```python
from build123d import *

# Parameters (mm, degrees)
F0_R         = 12.5
F0_R_2       = 10.9
F3_W         = 620
F3_H         = 800
F4_DEPTH     = 1.6
F5_R         = 15
F6_R         = 15
F7_W         = 558.6059093475
F7_H         = 742.6531389356
F8_DEPTH     = 15
F9_W         = 530.512617901
F9_H         = 715.3386492282
F10_DEPTH    = 15
F11_R        = 5
F12_T1_DEPTH = 10
F12_S5_W     = 5.1
F12_S5_H     = 5.1
F12_T6_DEPTH = 5.1


# Not quite as in the source:
# - a fillet or chamfer that OpenCascade refuses, or shapes differently, is made with other operations: its cross-section is extruded or revolved along the edge and cut away or added


with BuildPart() as f2:
    # F2: sweep along a path in F1
    with BuildLine(Plane.XZ) as f2_path:
        Line((0, 0), (0, 800))
        ThreePointArc((0, 800), (29.2893218813, 870.7106781187), (100, 900))
        Line((100, 900), (450, 900))
        ThreePointArc((450, 900), (520.7106781187, 870.7106781187), (550, 800))
        Line((550, 800), (550, 0))
    # F0 (on Top) → F2 (sweep)
    with BuildSketch(Plane.XY):
        Circle(F0_R)
        Circle(F0_R_2, mode=Mode.SUBTRACT)
    sweep(path=f2_path.line)

    # F3 (on Top) → F4 (join)
    with BuildSketch(Plane.XY):
        with Locations((276.0508990288, 338.4082295001)):
            Rectangle(F3_W, F3_H)
    extrude(amount=-F4_DEPTH)

    # F5
    f5_edges = [f2.edges().sort_by_distance(p)[0] for p in [
        (-33.949101, 738.40823, -0.8),
    ]]
    fillet(f5_edges, radius=F5_R)

    # F6
    f6_edges = [f2.edges().sort_by_distance(p)[0] for p in [
        (586.050899, 738.40823, -0.8),
    ]]
    fillet(f6_edges, radius=F6_R)

    # F7 (on face) → F8 (join)
    with BuildSketch(Plane(origin=(0, 0, -1.6), x_dir=(1, 0, 0), z_dir=(0, 0, -1))):
        with Locations((279.3029546738, -329.9668394029)):
            Rectangle(F7_W, F7_H)
    extrude(amount=F8_DEPTH)

    # F9 (on face) → F10 (cut)
    with BuildSketch(Plane(origin=(0, 0, -16.6), x_dir=(1, 0, 0), z_dir=(0, 0, -1))):
        with Locations((281.7520266399, -330.8358481154)):
            Rectangle(F9_W, F9_H)
    extrude(amount=-F10_DEPTH, mode=Mode.SUBTRACT)

    # F11
    f11_edges = [f2.edges().sort_by_distance(p)[0] for p in [
        (558.605909, 329.966839, -16.6),
        (547.008336, 330.835848, -16.6),
        (279.302955, -41.35973, -16.6),
        (281.752027, -26.833476, -16.6),
        (16.495718, 330.835848, -16.6),
        (0, 329.966839, -16.6),
        (281.752027, 688.505173, -16.6),
        (279.302955, 701.293409, -16.6),
        (558.605909, 701.293409, -9.1),
        (0, 701.293409, -9.1),
        (0, -41.35973, -9.1),
    ]]
    fillet(f11_edges, radius=F11_R)

    # F12: fillet of radius 5 on 2 edges, made by hand

    # F12_s2 → F12_t1 (cut)
    with BuildSketch(Plane.XY.offset(-11.6)):
        with BuildLine():
            ThreePointArc((558.6059093475, -36.3597300649), (557.1414432535, -39.8952639708), (553.6059093475, -41.3597300649))
            Line((553.6059093475, -41.3597300649), (558.6059093475, -41.3597300649))
            Line((558.6059093475, -41.3597300649), (558.6059093475, -36.3597300649))
        make_face()
    extrude(amount=F12_T1_DEPTH, mode=Mode.SUBTRACT)


with BuildPart() as f12_tool4:
    # F12_s5 → F12_t6 (new body)
    with BuildSketch(Plane.YZ.offset(553.6059093475)):
        with Locations((-38.9097300649, -14.15)):
            Rectangle(F12_S5_W, F12_S5_H)
    extrude(amount=F12_T6_DEPTH)

    # F12_s7 → F12_t8 (revolve, cut)
    with BuildSketch(Plane(origin=(553.6059093475, -36.3597300649, -11.6), x_dir=(0, 0.7071067812, 0.7071067812), z_dir=(0, 0.7071067812, -0.7071067812))):
        with BuildLine():
            ThreePointArc((0, -5), (5, 0), (0, 5))
            Line((0, 5), (0, -5))
        make_face()
    revolve(axis=Axis((553.6059093475, -36.3597300649, -11.6), (1, 0, 0)), mode=Mode.SUBTRACT)


with BuildPart() as f2_1:
    add(f2.part)

    # F12_t3: cut F12_tool4
    add(f12_tool4.part, mode=Mode.SUBTRACT)


solid = f2_1.part
```
The model under review builds one solid part; all positions refer to its coordinate system, in mm. A direction names the side the tool comes from. Round coordinates to 2 decimals unless told otherwise and drop trailing zeros. Loops run counter-clockwise (first coordinate to the right, second up) from the corner with the lowest first, then second, coordinate; pieces in that order, holes last. Notation, with made-up numbers: M 10.25,89.5 L 54.25,89.5 A14 cw 54.25,113.5 Z; hole C -24.5,80 d6. An arc over 180 degrees is marked long. Answer as a JSON object with one key per item and string values.
(1) To check wall thickness, follow line 1 along X through (y, z) = (1, 412); line 2 along Y through (x, z) = (0, 476.5); line 3 along X through (y, z) = (4, 30). State the ranges of each line that lie inside material, in increasing order.
Resolved:
{"line 1": "-12.46 to -10.85, 10.85 to 12.46, 537.54 to 539.15, 560.85 to 562.46", "line 2": "-12.5 to -10.9, 10.9 to 12.5", "line 3": "-11.84 to -10.14, 10.14 to 11.84, 538.16 to 539.86, 560.14 to 561.84"}
(2) Tool access review of faces 3 (the flat face through (-1, 340, -1.6)), 4 (the cylindrical face through (10.4, 3.27, 405.6)): name each direction out of +Z, -Z, +X, -X, +Y, -Y from which nothing blocks a thin tool from reaching the whole face with its end or side.
Resolved:
{"face 3": "-Z", "face 4": "none"}
(3) Draft analysis for pull direction Z (two halves, no side actions). For faces 1 (the cylindrical face through (11.923, 3.755, 405.6)), 2 (the flat face through (278, 326, -1.6)), state which applies: released by +Z, released by -Z, zero draft, split by the parting line, or undercut.
Resolved:
{"face 1": "undercut", "face 2": "released by -Z"}
(4) Take a section at B-B on z = 290. Give the boundary of the cut face in (x, y), and give its area (3 significant figures).
Resolved:
{"outline": "C 0,0 d25; C 550,0 d25; hole C 0,0 d21.8; hole C 550,0 d21.8", "area": "235 mm²"}
(5) Clearance check with flat-ended pins moving along their axes: P1, Ø6.5, axis at x = 547, y = -4, coming from the +Z side; P2, Ø3, axis at x = 316, z = -6, coming from the -Y side; P3, Ø3, axis at y = 222.5, z = -7.5, coming from the -X side. State where each tip first meets the part, or that it passes through.
Resolved:
{"P1": "z = 861.28", "P2": "y = -41.36", "P3": "x = 0"}
(6) Take a section at C-C on y = 297. Give the boundary of the cut face in (x, z).
Resolved:
{"outline": "M -33.95,-1.6 L 0,-1.6 L 0,-11.6 A5 ccw 5,-16.6 L 11.5,-16.6 A5 ccw 16.5,-11.6 L 16.5,-1.6 L 547.01,-1.6 L 547.01,-11.6 A5 ccw 552.01,-16.6 L 553.61,-16.6 A5 ccw 558.61,-11.6 L 558.61,-1.6 L 586.05,-1.6 L 586.05,0 L -33.95,0 Z"}
(7) Take a section at D-D on x = 504. Count the separate pieces of the cut face and the enclosed holes in it, and give its area (3 significant figures).
Resolved:
{"separate pieces": "2", "enclosed holes": "1", "area": "1,810 mm²"}
(8) Take a section at A-A on x = 208. Give the boundary of the cut face in (y, z).
Resolved:
{"outline": "M -61.59,-1.6 L -41.36,-1.6 L -41.36,-11.6 A5 ccw -36.36,-16.6 L -31.83,-16.6 A5 ccw -26.83,-11.6 L -26.83,-1.6 L 688.51,-1.6 L 688.51,-11.6 A5 ccw 693.51,-16.6 L 696.29,-16.6 A5 ccw 701.29,-11.6 L 701.29,-1.6 L 738.41,-1.6 L 738.41,0 L -61.59,0 Z; C 0,900 d25; hole C 0,900 d21.8"}
